Build history of the part. All positions in model axes, mm. A direction names the side the tool comes from. Round coordinates to 2 decimals unless told otherwise and drop trailing zeros. Write each loop counter-clockwise with the first axis right and the second up, starting at its lowest first coordinate (ties: lowest second). Pieces come first, ordered by that corner, then holes.
Item 1: Band-saw the part on A-A, the plane y = -278.5. Write the cut outline in (x, z), then the cut area to 3 significant figures.
Item 2: 3-axis set-ups, long thin cutter, end or side, ignore diameter. For faces 1 (the flat face through (-462, -284, 236.307)), 2 (the cylindrical face through (-464.297, -6.014, 252.918)): which of +Z, -Z, +X, -X, +Y, -Y reach the whole face in a straight line?
Item 3: Drop flat-ended pins along their axis: pin 1 Ø12 at (x, z) = (-233, 89) entering from -Y; pin 2 Ø6 at (x, y) = (-88.5, -508) entering from -Z; pin 3 Ø1.5 at (x, z) = (-53, 108) entering from -Y; pin 4 Ø3 at (x, z) = (-340.5, 117) entering from +Y. Give the stop position or say it passes through.
Item 4: Wall check: probe 1 along X at (y, z) = (-28.5, 225); probe 2 along Y at (x, z) = (-61, 202.5); probe 3 along X at (y, z) = (-225, 210.5). Give the ranges that are in metal, low to high.
Item 5: Band-saw the part on D-D, the plane z = 26.5. Write the cut outline in (x, y).
Item 6: Band-saw the part on B-B, the plane x = -266. Write the cut outline in (y, z), then the cut area to 3 significant figures.
Item 7: Band-saw the part on C-C, the plane z = 75. Write the cut outline in (x, y), then the cut area to 3 significant figures.
```python
from build123d import *

# Parameters (mm, degrees)
F1_DEPTH = 570
F3_DEPTH = 470.001
F4_R     = 20


with BuildPart() as f1:
    # F0 (on Front) → F1 (new body)
    with BuildSketch(Plane.XZ):
        with BuildLine():
            Line((-235, 0), (-35, 0))
            Line((-35, 0), (-20, 236.3072186708))
            Line((-20, 236.3072186708), (0, 236.3072186708))
            Line((0, 236.3072186708), (0, 270))
            ThreePointArc((0, 270), (-5.8578643763, 284.1421356237), (-20, 290))
            Line((-20, 290), (-235, 290))
            Line((-235, 290), (-235, 0))
        make_face()
        with BuildLine():
            Line((-435, 0), (-235, 0))
            Line((-235, 0), (-235, 290))
            Line((-235, 290), (-450, 290))
            ThreePointArc((-450, 290), (-464.1421356237, 284.1421356237), (-470, 270))
            Line((-470, 270), (-470, 236.3072186708))
            Line((-470, 236.3072186708), (-450, 236.3072186708))
            Line((-450, 236.3072186708), (-435, 0))
        make_face()
    extrude(amount=F1_DEPTH)

    # F2 (on Right) → F3 (cut, through all)
    with BuildSketch(Plane.YZ):
        Polygon((-50, 0), (0, 0), (0, 236.3072186708), (-20, 236.3072186708), align=None)
        Polygon((-570, 0), (-520, 0), (-550, 236.3072186708), (-570, 236.3072186708), align=None)
    extrude(amount=-F3_DEPTH, mode=Mode.SUBTRACT)

    # F4
    f4_edges = [f1.edges().sort_by_distance(p)[0] for p in [
        (-235, -570, 290),
        (-235, 0, 290),
    ]]
    fillet(f4_edges, radius=F4_R)


solid = f1.part
```
Results:
1. outline: (-470, 236.31) - (-450, 236.31) - (-435, 0) - (-35, 0) - (-20, 236.31) - (0, 236.31) - (0, 270) arc R20 ccw to (-20, 290) - (-450, 290) arc R20 ccw to (-470, 270) - close
1. area: 123,000 mm2
2. face 1: -Z
2. face 2: +Z, -Z, -X, +Y
3. pin 1: stops at y = -532.06
3. pin 2: stops at z = 0
3. pin 3: stops at y = -533.81
3. pin 4: stops at y = -34.96
4. probe 1: x = -449.28 to -20.72
4. probe 2: y = -545.71 to -24.29
4. probe 3: x = -448.36 to -21.64
5. outline: (-436.68, -523.36) - (-33.32, -523.36) - (-33.32, -46.64) - (-436.68, -46.64) - close
6. outline: (-570, 236.31) - (-550, 236.31) - (-520, 0) - (-50, 0) - (-20, 236.31) - (0, 236.31) - (0, 270) arc R20 ccw to (-20, 290) - (-550, 290) arc R20 ccw to (-570, 270) - close
6. area: 149,000 mm2
7. outline: (-439.76, -529.52) - (-30.24, -529.52) - (-30.24, -40.48) - (-439.76, -40.48) - close
7. area: 200,000 mm2
